Autodesk Inventor part; units mm, degrees
ref_plane "YZ Plane" through (0, 0, 0) normal (1, 0, 0) x (0, 1, 0)
ref_plane "XZ Plane" through (0, 0, 0) normal (0, 1, 0) x (-1, 0, 0)
ref_plane "XY Plane" through (0, 0, 0) normal (0, 0, 1) x (1, 0, 0)
sketch "Sketch1" plane through (0, 0, 0) normal (0, 0, 1) x (1, 0, 0)
  line L0 (0, 0) -> (-42.672, 0)
  line L1 (-42.672, 0) -> (-42.672, 40)
  line L2 (-42.672, 40) -> (0, 40)
  line L3 (0, 40) -> (0, 0)
  dimension "d0" = 42.672
  dimension "d1" = 40
extrude "Extrusion1" add sketch "Sketch1" along normal blind 6.35
sketch "Sketch2" plane through (0, 0, 6.35) normal (0, 0, 1) x (1, 0, 0)
  line L0 (-42.672, 0) -> (0, 0)
  line L1 (-42.672, 40) -> (-36.322, 40)
  line L2 (-36.322, 40) -> (-36.322, 0)
  line L3 (-36.322, 0) -> (-42.672, 0)
  line L4 (-42.672, 0) -> (-42.672, 40)
  dimension "d4" = 6.35
extrude "Extrusion2" add sketch "Sketch2" along normal blind 25.4
sketch "Sketch3" plane through (0, 0, 6.35) normal (0, 0, 1) x (1, 0, 0)
  line L0 (-36.322, 0) -> (0, 0)
  line L1 (0, 40) -> (-6.35, 40)
  line L2 (-6.35, 40) -> (-6.35, 0)
  line L3 (-6.35, 0) -> (0, 0)
  line L4 (0, 0) -> (0, 40)
  dimension "d7" = 6.35
extrude "Extrusion3" add sketch "Sketch3" along normal blind 25.4
sketch "Sketch4" plane through (0, 0, 0) normal (1, 0, 0) x (0, 0, -1)
  circle A0 centre (-24.4119, 20) radius 2.413
  dimension "d10" = 4.826
extrude "Extrusion4" cut sketch "Sketch4" against normal blind 76.2
sketch "Sketch5" plane through (0, 0, 6.35) normal (0, 0, 1) x (1, 0, 0)
  line L0 (-6.35, 40) -> (-36.322, 40)
  line L1 (-36.322, 0) -> (-6.35, 0)
  point P0 (0, 0)
  point P1 (-21.336, 33.904)
  point P2 (-21.336, 6.096)
  dimension "d13" = 6.096
  dimension "d14" = 6.096
hole "Hole1" at (-21.336, 33.904, 6.35) at (-21.336, 6.096, 6.35) direction (0, 0, -1) diameter 5 end through all
properties part number "LiftBase2" material "Aluminum 6061"
Here's how the part is built. I have some questions about the finished solid (model axes, mm). A direction names the side the tool comes from. Coordinates: 2 decimals unless noted, no trailing zeros. Write each loop counter-clockwise with the first axis right and the second up, starting at its lowest first coordinate (ties: lowest second). Pieces come first, ordered by that corner, then holes. Notation, with made-up numbers: (47, 23.5) - (98, 23.5) arc R31 cw to (98, 61.5) - close; hole circle Ø4 at (-19, 54). An arc over 180 degrees is marked (long way). One line per item, written item: value.
1) I need wall thicknesses on line 1 along X through (y, z) = (35.5, 23); line 2 along Y through (x, z) = (-23, 5.5); line 3 along Z through (x, y) = (-31, 35). Which ranges of each line are inside material? Lowest first, please.
Model answer:
line 1: x = -42.67 to -36.32, -6.35 to 0
line 2: y = 0 to 4.23, 7.96 to 32.04, 35.77 to 40
line 3: z = 0 to 6.35
2) On a 3-axis mill with a long thin cutter (end or side, diameter ignored), from which of +Z, -Z, +X, -X, +Y, -Y can I reach the whole of each face in a straight line? I mean faces 1 (the flat face through (-36.322, 20, 19)), 2 (the cylindrical face through (-18.895, 34.446, 3.131)). Say none if no direction works.
Model answer:
face 1: +Z, +Y, -Y
face 2: +Z, -Z
3) Suppose I cut it at A-A on y = 20. Write out the boundary of the cut face in (x, z), and give its area (3 significant figures).
Model answer:
outline: (-42.67, 0) - (0, 0) - (0, 22) - (-6.35, 22) - (-6.35, 6.35) - (-36.32, 6.35) - (-36.32, 22) - (-42.67, 22) - close; (-42.67, 26.82) - (-36.32, 26.82) - (-36.32, 31.75) - (-42.67, 31.75) - close; (-6.35, 26.82) - (0, 26.82) - (0, 31.75) - (-6.35, 31.75) - close
area: 532 mm²
4) We'd pull the mould along Y, two halves only. Please class faces 3 (the flat face through (-22, 0, 5)), 4 (the flat face through (-40, 20, 31.75)), 5 (the cylindrical face through (-39.453, 17.644, 24.935)), 6 (the flat face through (-21, 40, 5)): pulls with the +Y half, pulls with the -Y half, needs draft (parallel to the pull), parting line crosses it, or undercut.
Model answer:
face 3: pulls with the -Y half
face 4: needs draft
face 5: undercut
face 6: pulls with the +Y half
5) Suppose I cut it at D-D on x = -9. Write out the boundary of the cut face in (y, z), and give its area (3 significant figures).
Model answer:
outline: (0, 0) - (40, 0) - (40, 6.35) - (0, 6.35) - close
area: 254 mm²
6) Suppose I cut it at C-C on y = 5. Write out the boundary of the cut face in (x, z), and give its area (3 significant figures).
Model answer:
outline: (-42.67, 0) - (-23.58, 0) - (-23.58, 6.35) - (-36.32, 6.35) - (-36.32, 31.75) - (-42.67, 31.75) - close; (-19.09, 0) - (0, 0) - (0, 31.75) - (-6.35, 31.75) - (-6.35, 6.35) - (-19.09, 6.35) - close
area: 565 mm²
7) Suppose I cut it at B-B on y = 37. Write out the boundary of the cut face in (x, z), and give its area (3 significant figures).
Model answer:
outline: (-42.67, 0) - (0, 0) - (0, 31.75) - (-6.35, 31.75) - (-6.35, 6.35) - (-36.32, 6.35) - (-36.32, 31.75) - (-42.67, 31.75) - close
area: 594 mm²
